Verification items for this drawing (mm, ordinates from the low corner). Coordinates: 2 decimals unless noted, no trailing zeros. Order: outer loops, then holes, each group sorted by start corner. A loop starts at its lowest first (then second) coordinate and runs counter-clockwise, first axis right, second up. Notation, with made-up numbers: (-29, -1.75) -> (14, -1.75) arc R12 ccw to (14, 16.25) -> close; hole circle Ø3 at (81, -7). An arc over 180 degrees is marked (long way). Write item = value, one per line. Start each with the question number.
1. Go/stop test with flat-tipped pins: P1, Ø1.5, axis at x = 51.5, y = 55.5, coming from the +Z side; P2, Ø3, axis at y = 77.5, z = 9.5, coming from the +X side; P3, Ø5, axis at y = 24, z = 23.5, coming from the +X side. Record where each tip stops, or that it passes through.
2. Cross-section at D-D on z = 27.25. Record the cut outline in (x, y).
3. Cross-section at B-B on x = 50. Record the cut outline in (y, z), plus the area to 3 significant figures.
4. Cross-section at A-A on z = 9. Record the cut outline in (x, y), plus the area to 3 significant figures.
5. Release check for a two-part mould opening along Y. For the marked faces 1, 2 and 3 record: +Y half, -Y half, draft (parallel to the pull), parting line (faces both ways), or undercut.
6. Thickness scan on line 1 along Y through (x, z) = (50, 15.75); line 2 along Y through (x, z) = (50, 21.75); line 3 along Z through (x, y) = (50.5, 59.5). Record the ranges inside material, lowest first. Write a range as from..to.
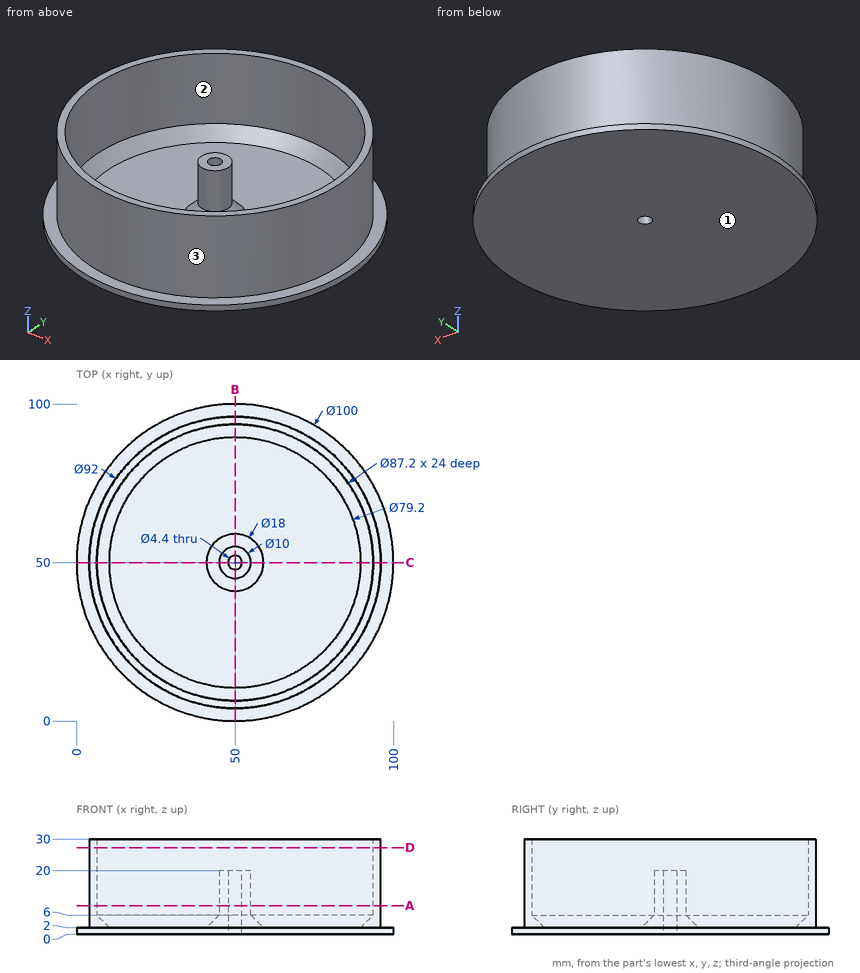
Worked out:
q1.P1 = 20
q1.P2 = 87.95
q1.P3 = 89.54
q2.outline = circle Ø92 at (50, 50); hole circle Ø87.2 at (50, 50)
q3.outline = (0, 0) -> (47.8, 0) -> (47.8, 20) -> (45, 20) -> (45, 6) -> (41, 2) -> (10.4, 2) -> (6.4, 6) -> (6.4, 30) -> (4, 30) -> (4, 2) -> (0, 2) -> close; (52.2, 0) -> (100, 0) -> (100, 2) -> (96, 2) -> (96, 30) -> (93.6, 30) -> (93.6, 6) -> (89.6, 2) -> (59, 2) -> (55, 6) -> (55, 20) -> (52.2, 20) -> close
q3.area = 458 mm²
q4.outline = circle Ø92 at (50, 50); circle Ø10 at (50, 50); hole circle Ø87.2 at (50, 50); hole circle Ø4.4 at (50, 50)
q4.area = 739 mm²
q5.face_1 = draft
q5.face_2 = undercut
q5.face_3 = parting line
q6.line_1 = 4..6.4, 45..47.8, 52.2..55, 93.6..96
q6.line_2 = 4..6.4, 93.6..96
q6.line_3 = 0..2
